```python
from build123d import *

# Parameters (mm, degrees)
SKETCH1_W           = 130.175
SKETCH1_H           = 19.05
BOSS_EXTRUDE1_DEPTH = 19.05
SKETCH2_W           = 3.175
SKETCH2_H           = 38.1
BOSS_EXTRUDE2_DEPTH = 130.175
SKETCH4_R           = 1.190625
CUT_EXTRUDE1_DEPTH  = 4.175
SKETCH5_W           = 15.875
SKETCH5_H           = 101.6
CUT_EXTRUDE2_DEPTH  = 39.1


with BuildPart() as part:
    # Sketch1 → Boss-Extrude1 (new body)
    with BuildSketch(Plane(origin=(0, 0, 0), x_dir=(0, 0, -1), z_dir=(1, 0, 0))):
        Rectangle(SKETCH1_W, SKETCH1_H)
    extrude(amount=BOSS_EXTRUDE1_DEPTH)

    # Sketch2 → Boss-Extrude2 (add)
    with BuildSketch(Plane.XY.offset(65.0875)):
        with Locations((1.5875, 0)):
            Rectangle(SKETCH2_W, SKETCH2_H)
    extrude(amount=-BOSS_EXTRUDE2_DEPTH)

    # Sketch4 → Cut-Extrude1 (cut, through all)
    with BuildSketch(Plane(origin=(3.175, 0, 0), x_dir=(0, 0, -1), z_dir=(1, 0, 0))):
        with Locations((-58.7375, -14.2875)):
            Circle(SKETCH4_R)
        with Locations((58.7375, -14.2875)):
            Circle(SKETCH4_R)
        with Locations((58.7375, 14.2875)):
            Circle(SKETCH4_R)
        with Locations((-58.7375, 14.2875)):
            Circle(SKETCH4_R)
    extrude(amount=-CUT_EXTRUDE1_DEPTH, mode=Mode.SUBTRACT)

    # Sketch5 → Cut-Extrude2 (cut, through all)
    with BuildSketch(Plane(origin=(0, -19.05, 0), x_dir=(-1, 0, 0), z_dir=(0, -1, 0))):
        with Locations((-7.9375, 0)):
            Rectangle(SKETCH5_W, SKETCH5_H)
    extrude(amount=-CUT_EXTRUDE2_DEPTH, mode=Mode.SUBTRACT)


solid = part.part
```
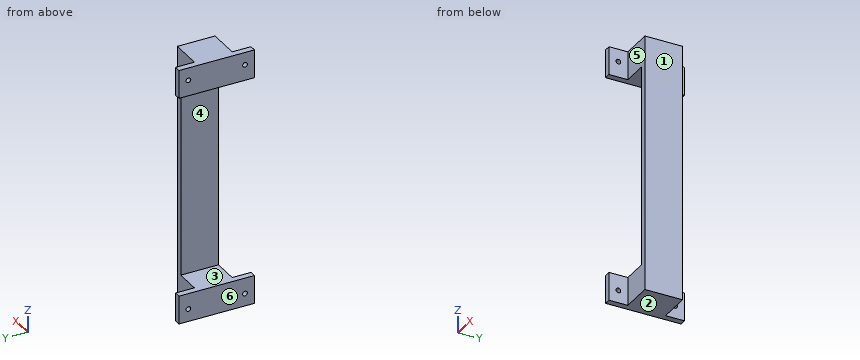
CAD build for the part. Positions are in the model's coordinates, mm. Face numbers are marked on the shaded views. A direction names the side the tool comes from. Round coordinates to 2 decimals unless told otherwise and drop trailing zeros. Order: outer loops, then holes, each group sorted by start corner. A loop starts at its lowest first (then second) coordinate and runs counter-clockwise, first axis right, second up.
Item 1: Saw through at C-C on x = 7.25. Write the cut outline in (y, z) (1 decimal).
Item 2: Probe line 1 along Z through (x, y) = (9.5, 8.5); line 2 along X through (y, z) = (5.5, -14) (3 decimals); line 3 along Y through (x, z) = (14.5, 54) (3 decimals). List the from-to ranges inside material, lowest first.
Item 3: Saw through at D-D on z = 4. Write the cut outline in (x, y) (3 decimals).
Item 4: Mould opens along Z. For the marked faces 1, 2 and 3 say: pulls with the +Z half, pulls with the -Z half, needs draft (parallel to the pull), parting line crosses it, or undercut.
Item 5: Saw through at A-A on x = 1.75. Write the cut outline in (y, z).
Item 6: Pin check, flat tips, straight feed: pin 1 (15 mm diameter, centred on y = -2, z = 9, fed in from -X) (3 decimals); pin 2 (5 mm diameter, centred on x = 13.5, z = -29, fed in from -Y) (3 decimals); pin 3 (7.5 mm diameter, centred on y = -16.5, z = -59.5, fed in from +X) (3 decimals). Stop position of each tip, or through.
Item 7: Tool access for the marked faces 4, 5 and 6: list every direction of +Z, -Z, +X, -X, +Y, -Y with a clear straight run to the whole face (end or side of a thin tool).
Item 8: Saw through at B-B on y = -12. Write the cut outline in (x, z) (1 decimal), then the cut area to 3 significant figures.
Reported:
1. outline: (-9.5, -65.1) - (9.5, -65.1) - (9.5, -50.8) - (-9.5, -50.8) - close; (-9.5, 50.8) - (9.5, 50.8) - (9.5, 65.1) - (-9.5, 65.1) - close
2. line 1: z = -65.09 to -50.8, 50.8 to 65.09
2. line 2: x = 15.875 to 19.05
2. line 3: y = -9.525 to 9.525
3. outline: (15.875, -9.525) - (19.05, -9.525) - (19.05, 9.525) - (15.875, 9.525) - close
4. face 1: needs draft
4. face 2: pulls with the -Z half
4. face 3: undercut
5. outline: (-19.05, -65.09) - (19.05, -65.09) - (19.05, -50.8) - (-19.05, -50.8) - close; (-19.05, 50.8) - (19.05, 50.8) - (19.05, 65.09) - (-19.05, 65.09) - close; hole circle Ø2.38 at (-14.29, -58.74); hole circle Ø2.38 at (-14.29, 58.74); hole circle Ø2.38 at (14.29, -58.74); hole circle Ø2.38 at (14.29, 58.74)
6. pin 1: stops at x = 15.875
6. pin 2: stops at y = -9.525
6. pin 3: stops at x = 3.175
7. face 4: -X, +Y, -Y
7. face 5: +Z, -Z, +X, -Y
7. face 6: +Z, -Z, -X, +Y, -Y
8. outline: (0, -65.1) - (3.2, -65.1) - (3.2, -50.8) - (0, -50.8) - close; (0, 50.8) - (3.2, 50.8) - (3.2, 65.1) - (0, 65.1) - close
8. area: 90.7 mm2
